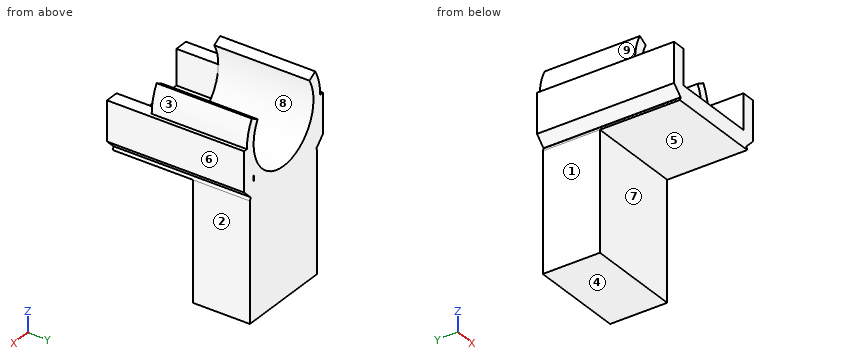
Autodesk Inventor part; units mm, degrees
ref_plane "YZ Plane" through (0, 0, 0) normal (1, 0, 0) x (0, 1, 0)
ref_plane "XZ Plane" through (0, 0, 0) normal (0, 1, 0) x (-1, 0, 0)
ref_plane "XY Plane" through (0, 0, 0) normal (0, 0, 1) x (1, 0, 0)
sketch "Sketch1" plane through (0, 0, 0) normal (0, 1, 0) x (-1, 0, 0)
  line L0 (0, 0) -> (15, 0)
  line L1 (15, 0) -> (15, 34)
  line L2 (15, 34) -> (0, 34)
  line L3 (0, 34) -> (0, 0)
  line L4 (7.5, 34) -> (7.5, 36.5)
  line L5 (7.5, 36.5) -> (7.5, 47.61)
  circle A0 centre (7.5, 47.61) radius 11.11
  circle A1 centre (7.5, 47.61) radius 13.61
  line L6 (7.5, 47.61) -> (19.2866, 54.415)
  line L7 (7.5, 47.61) -> (21.11, 47.61) construction
  line L8 (7.5, 47.61) -> (-4.2866, 54.415)
  line L9 (7.5, 47.61) -> (21.11, 47.61) construction
  line L10 (15, 34) -> (18.5355, 37.5355)
  line L11 (15, 34) -> (20, 34) construction
  line L12 (18.5355, 37.5355) -> (18.5355, 39.6445)
  line L13 (0, 34) -> (-3.5355, 37.5355)
  line L14 (-3.5355, 37.5355) -> (-3.5355, 39.6445)
  line L15 (7.5, 47.61) -> (7.5, 56.86)
  line L16 (7.5, 56.86) -> (17.4835, 56.86)
  line L17 (7.5, 56.86) -> (-2.4835, 56.86)
  line L18 (7.5, 47.61) -> (-6.11, 47.61)
  line L19 (7.5, 47.61) -> (7.5, 38.36)
  line L20 (7.5, 38.36) -> (17.4835, 38.36)
  line L21 (7.5, 38.36) -> (-2.4835, 38.36)
  line L22 (7.5, 38.36) -> (-3.61, 38.36)
  line L23 (-3.61, 38.36) -> (-3.61, 47.61)
  line L24 (-3.61, 47.61) -> (-3.61, 56.86)
  line L25 (-3.61, 56.86) -> (-2.4835, 56.86)
  line L26 (7.5, 56.86) -> (18.61, 56.86)
  line L27 (18.61, 56.86) -> (18.61, 47.61)
  line L28 (7.5, 38.36) -> (18.61, 38.36)
  line L29 (18.61, 38.36) -> (18.61, 47.61)
  line L30 (7.5, 0) -> (7.5, 3)
  line L31 (7.5, 3) -> (0, 3)
  line L32 (7.5, 3) -> (15, 3)
  line L33 (7.5, 3) -> (20, 3)
  line L34 (7.5, 3) -> (-5, 3)
  line L35 (7.5, 34) -> (20, 34)
  line L36 (7.5, 34) -> (-5, 34)
  line L37 (-5, 34) -> (-5, 3)
  line L38 (20, 3) -> (20, 34)
  line L39 (18.61, 38.36) -> (22.1455, 34.8245)
  line L40 (-3.61, 56.86) -> (-7.1455, 60.3955)
  line L41 (22.1455, 34.8245) -> (-7.1455, 34.8245)
  line L42 (-7.1455, 34.8245) -> (-7.1455, 60.3955)
  line L43 (-7.1455, 60.3955) -> (22.1455, 60.3955)
  line L44 (22.1455, 60.3955) -> (22.1455, 34.8245)
  line L45 (-3.5355, 37.5355) -> (-5, 34)
  line L46 (18.5355, 37.5355) -> (20, 34)
  line L47 (7.5, 47.61) -> (-7.1455, 47.61)
  line L48 (7.5, 47.61) -> (22.1455, 47.61)
  point P0 (17.1215, 53.165)
  point P1 (-2.1215, 53.165)
  point P2 (0, 34)
  point P3 (0, 3)
  point P4 (0, 34)
  point P5 (2.835, 60.3955)
  point P6 (-4.6585, 34.8245)
  point P7 (-3.5355, 38.36)
  point P8 (-3.61, 39.7487)
  point P9 (-3.61, 55.4713)
  point P10 (12.165, 60.3955)
  point P11 (18.61, 55.4713)
  point P12 (18.61, 39.7487)
  point P13 (18.5355, 38.36)
  point P14 (19.6585, 34.8245)
  point P15 (18.61, 47.61)
  dimension "d0" = 15
  dimension "d1" = 34
  dimension "d2" = 2.5
  dimension "d3" = 11.11
  dimension "d4" = 30
  dimension "d5" = 150
  dimension "d6" = 5
  dimension "d7" = 45
  dimension "d10" = 9.25
  dimension "d11" = 11.11
  dimension "d12" = 11.11
  dimension "d13" = 11.11
  dimension "d14" = 3
  dimension "d15" = 12.5
  dimension "d16" = 5
  dimension "d17" = 5
extrude "Extrusion1" add sketch "Sketch1" along normal blind 15 and the other way blind 10 contours L13 L41 A1 L2 | L36 L45 L41 L13 | A1 L41 L10 L2 | A1 L41 L4 | L4 L41 A1 | L41 L45 L13 | L13 L14 L22 A1 L41 | L10 L41 L46 L35 | L41 A1 L21 A0 L4 | L4 A0 L20 A1 L41 | A1 L28 L12 L10 L41 | L45 L41 L42 L47 A1 L23 L22 L14 | L10 L46 L41 | L22 L14 A1 | A1 L23 A0 L21 | L20 A0 L29 A1 | A1 L12 L28 | L12 L28 L39 L41 L46 | L39 L29 A1 L48 L44 | L24 L8 A0 | L23 A1 L18 | L18 A1 L8 L24 | A0 L6 L27 | L48 A1 L29 | L27 L6 A1 L48
extrude "Extrusion2" add sketch "Sketch1" along normal blind 15 contours L34 L37 L36 L3 | L3 L2 L1 L32 L31 | L1 L35 L38 L33
extrude "Extrusion3" add sketch "Sketch1" against normal blind 11 from surface at -10 contours L13 L41 A1 L2 | L36 L45 L41 L13 | A1 L41 L10 L2 | A1 L41 L4 | L4 L41 A1 | L41 L45 L13 | L13 L14 L22 A1 L41 | L10 L41 L46 L35 | L41 A1 L21 A0 L4 | L4 A0 L20 A1 L41 | A1 L28 L12 L10 L41 | L45 L41 L42 L47 A1 L23 L22 L14 | L10 L46 L41 | A0 L21 L5 | L5 L20 A0 | L12 L28 L39 L41 L46 | L39 L29 A1 L48 L44 | L23 A1 L18 | L48 A1 L29
chamfer "Chamfer2" distance 2.4 angle 45 2 edges at (7.1455, -3, 34.8245) (-22.1455, -3, 34.8245)
properties part number "motor holder v2"
Can you work these out from the model? Positions are in its coordinate system, mm. Face numbers are marked on the shaded views. A direction names the side the tool comes from. Round coordinates to 2 decimals unless told otherwise and drop trailing zeros. Loops run counter-clockwise (first coordinate to the right, second up) from the corner with the lowest first, then second, coordinate; pieces in that order, holes last. Notation, with made-up numbers: M -14.75,40.25 L -7.75,40.25 A24 ccw -7.75,70.25 Z; hole C -27,37 d5. An arc over 180 degrees is marked long. Write item = value, one per line. Start each with the question number.
(1) Suppose I cut it at B-B on y = -12. Write out the boundary of the cut face in (x, z).
(2) Suppose I cut it at A-A on z = 43. Write out the boundary of the cut face in (x, y).
(3) Suppose I cut it at C-C on x = -7.5. Write out the boundary of the cut face in (y, z), plus the area to 3 significant figures.
(4) I'm going to push flat-ended pins straight in: P1, Ø1.5, axis at y = 4.5, z = 23, coming from the -X side; P2, Ø4.5, axis at y = 9.5, z = 14.5, coming from the +X side; P3, Ø4, axis at x = -12.5, y = 3, coming from the +Z side; P4, Ø1.5, axis at x = -17, z = 45, coming from the -Y side. Where does each tip first touch, or does it pass through?
(5) Suppose I cut it at D-D on y = 11. Give the number of separate pieces and of enclosed holes in the cut face, plus the area to 3 significant figures.
(6) Which directions (+Z, -Z, +X, -X, +Y, -Y) give clear straight access to the entire face, cutting with the end or side of a thin tool? Please do the marked faces 1, 2, 3, 4 and 5.
(7) If we mould it in two halves opening along X, with no side actions, what happens to the marked faces 6, 7, 8 and 9? For each: released by +X, released by -X, zero draft, split by the parting line, or undercut.
(8) I need wall thicknesses on line 1 along Z through (x, y) = (-14.75, -14.5); line 2 along Y through (x, z) = (-3.25, 12); line 3 along X through (y, z) = (7, 26.5). Which ranges of each line are inside material? Lowest first, please.
Answer block:
q1.outline = M -22.15,37.22 L -19.75,34.82 L -19.66,34.82 L -20,34 L 5,34 L 4.66,34.82 L 4.75,34.82 L 7.15,37.22 L 7.15,47.61 L 3.61,47.61 L 3.61,38.36 L -18.61,38.36 L -18.61,47.61 L -22.15,47.61 Z
q2.outline = M -22.15,-21 L -18.61,-21 L -18.61,-10 L -17.61,-10 L -17.61,15 L -22.15,15 Z; M 2.61,-10 L 3.61,-10 L 3.61,-21 L 7.15,-21 L 7.15,15 L 2.61,15 Z
q3.outline = M -21,34 L 0,34 L 0,3 L 15,3 L 15,36.5 L -10,36.5 L -10,38.36 L -21,38.36 Z
q3.area = 575 mm²
q4.P1 = -20
q4.P2 = 5
q4.P3 = 38.98
q4.P4 = through
q5.separate_pieces = 1
q5.enclosed_holes = 2
q5.area = 1,000 mm²
q6.face_1 = -Z, -X, +Y, -Y
q6.face_2 = -Z, +X, +Y, -Y
q6.face_3 = +Z, +X, +Y, -Y
q6.face_4 = -Z, +X, -X, +Y, -Y
q6.face_5 = -Z, +X, -X, -Y
q7.face_6 = released by +X
q7.face_7 = zero draft
q7.face_8 = undercut
q7.face_9 = released by -X
q8.line_1 = 34 to 38.36
q8.line_2 = 0 to 15
q8.line_3 = -20 to 5
